from build123d import *

# Parameters (mm, degrees)
SKETCH_1_W             = 528
SKETCH_1_H             = 326
EXTRUDE_1_DEPTH        = 16
SKETCH_2_W             = 528
SKETCH_2_H             = 16
EXTRUDE_2_DEPTH        = 40
EXTRUDE_3_DEPTH        = 528
EXTRUDE_4_DEPTH        = 12
PATTERN_LINEAR_1_COUNT = 2
PATTERN_LINEAR_1_PITCH = 112
SKETCH_5_W             = 100
SKETCH_5_H             = 12
EXTRUDE_5_DEPTH        = 123
SKETCH_6_W             = 100
SKETCH_6_H             = 12
EXTRUDE_6_DEPTH        = 100
MIRROR_2_COPY_1_DEPTH  = 12


with BuildPart() as part:
    # 草图1 → 凸台-拉伸1 (new body)
    with BuildSketch(Plane(origin=(0, 0, 0), x_dir=(1, 0, 0), z_dir=(0, 1, 0))):
        Rectangle(SKETCH_1_W, SKETCH_1_H)
    extrude(amount=EXTRUDE_1_DEPTH)

    # 草图2 → 凸台-拉伸2 (add)
    with BuildSketch(Plane.XZ):
        with Locations((0, 145)):
            Rectangle(SKETCH_2_W, SKETCH_2_H)
        with Locations((0, -145)):
            Rectangle(SKETCH_2_W, SKETCH_2_H)
    extrude(amount=EXTRUDE_2_DEPTH)

    # 草图3 → 凸台-拉伸3 (add)
    with BuildSketch(Plane(origin=(264, 0, 0), x_dir=(0, 0, -1), z_dir=(1, 0, 0))):
        Polygon((-137, -40), (-137, 0), (137, 0), (137, -40), (132, -40), (132, -5), (-132, -5), (-132, -40), align=None)
    extrude(amount=-EXTRUDE_3_DEPTH)

    # 草图4 → 凸台-拉伸4 (add)
    with BuildSketch(Plane.ZY.offset(264)):
        with BuildLine():
            Line((-70, 139), (70, 139))
            ThreePointArc((70, 139), (91.213203436, 130.213203436), (100, 109))
            Line((100, 109), (100, 16))
            Line((100, 16), (-100, 16))
            Line((-100, 16), (-100, 109))
            ThreePointArc((-100, 109), (-91.213203436, 130.213203436), (-70, 139))
        make_face()
    extrude_4 = extrude(amount=-EXTRUDE_4_DEPTH)

    # 阵列(线性)1: 凸台-拉伸4 ×2
    with Locations(*[(i * PATTERN_LINEAR_1_PITCH, 0, 0) for i in range(1, PATTERN_LINEAR_1_COUNT)]):
        add(extrude_4)

    # 草图5 → 凸台-拉伸5 (add)
    with BuildSketch(Plane(origin=(0, 16, 0), x_dir=(1, 0, 0), z_dir=(0, 1, 0))):
        with Locations((-202, 56)):
            Rectangle(SKETCH_5_W, SKETCH_5_H)
        with Locations((-202, -56)):
            Rectangle(SKETCH_5_W, SKETCH_5_H)
    extrude_5 = extrude(amount=EXTRUDE_5_DEPTH)

    # 草图6 → 凸台-拉伸6 (add)
    with BuildSketch(Plane.ZY.offset(152)):
        with Locations((0, 89)):
            Rectangle(SKETCH_6_W, SKETCH_6_H)
    extrude_6 = extrude(amount=EXTRUDE_6_DEPTH)

    # 镜向2: 凸台-拉伸4, 凸台-拉伸5, 凸台-拉伸6 across plane
    add(extrude_4.mirror(Plane(origin=(0, 0, 0), x_dir=(0, 0, 1), z_dir=(1, 0, 0))))
    add(extrude_5.mirror(Plane(origin=(0, 0, 0), x_dir=(0, 0, 1), z_dir=(1, 0, 0))))
    add(extrude_6.mirror(Plane(origin=(0, 0, 0), x_dir=(0, 0, 1), z_dir=(1, 0, 0))))

    # 镜向2 copy 1 sketch → 镜向2 copy 1 (add)
    with BuildSketch(Plane(origin=(152, 0, 0), x_dir=(0, 0, 1), z_dir=(1, 0, 0))):
        with BuildLine():
            Line((-70, -139), (70, -139))
            ThreePointArc((70, -139), (91.213203436, -130.213203436), (100, -109))
            Line((100, -109), (100, -16))
            Line((100, -16), (-100, -16))
            Line((-100, -16), (-100, -109))
            ThreePointArc((-100, -109), (-91.213203436, -130.213203436), (-70, -139))
        make_face()
    extrude(amount=-MIRROR_2_COPY_1_DEPTH)


solid = part.part
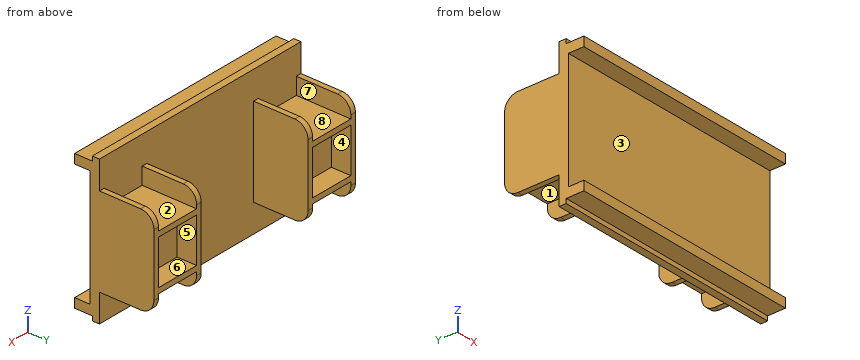
Verification items for the finished model (mm, model axes). Face numbers are marked on the shaded views. A direction names the side the tool comes from. Coordinates: 2 decimals unless noted, no trailing zeros. Order: outer loops, then holes, each group sorted by start corner. A loop starts at its lowest first (then second) coordinate and runs counter-clockwise, first axis right, second up. Notation, with made-up numbers: M -25.5,39.25 L 32.5,39.25 A6 cw 32.5,45.25 Z; hole C -27.5,-34 d3. An arc over 180 degrees is marked long. One line per item, written item: value. Start each with the question number.
Item 1: Depth check by flat-ended pin: P1, Ø10, axis at x = -14, z = -103.5, coming from the -Y side; P2, Ø1, axis at x = -154.5, y = 71, coming from the +Z side; P3, Ø6, axis at x = 256.5, y = 84, coming from the +Z side. Enter the tip coordinate at first touch or a pass-through.
Item 2: Thickness scan on probe 1 along X at (y, z) = (49, -69.5); probe 2 along X at (y, z) = (91, 39); probe 3 along Z at (x, y) = (15, -14). Record the ranges inside material, lowest first.
Item 3: Sectioned sample at D-D on x = -221.5. Record the cut outline in (y, z), then the cut area to 3 significant figures.
Item 4: Sectioned sample at B-B on y = -15.5. Record the cut outline in (x, z), then the cut area to 3 significant figures.
Item 5: Access from +Z, -Z, +X, -X, +Y, -Y to the whole of each face (thin tool, end or side, straight path). Record for the marked faces 1, 2, 3 and 4.
Item 6: Mould release check, pull along Z, two halves, no side actions. Record for the marked faces 5, 6, 7 and 8: pulls with the +Z half, pulls with the -Z half, needs draft (parallel to the pull), parting line crosses it, or undercut.
Item 7: Sectioned sample at A-A on y = 55.5. Give the number of separate pieces and of enclosed holes in the cut face, then the cut area to 3 significant figures.
Item 8: Sectioned sample at C-C on z = 15. Record the cut outline in (x, y), then the cut area to 3 significant figures.
Calculated:
1. P1: y = -5
1. P2: z = 62
1. P3: z = 100
2. probe 1: -264 to -252, -152 to -140, 140 to 152, 252 to 264
2. probe 2: -264 to -140, 140 to 264
2. probe 3: -153 to -132, 132 to 153
3. outline: M -40,-153 L 0,-153 L 0,-163 L 16,-163 L 16,-62 L 139,-62 L 139,-50 L 95,-50 L 95,50 L 139,50 L 139,62 L 16,62 L 16,163 L 0,163 L 0,153 L -40,153 L -40,132 L -5,132 L -5,-132 L -40,-132 Z; hole M 16,-50 L 83,-50 L 83,50 L 16,50 Z
3. area: 12,400 mm^2
4. outline: M -264,-153 L 264,-153 L 264,-132 L -264,-132 Z; M -264,132 L 264,132 L 264,153 L -264,153 Z
4. area: 22,200 mm^2
5. face 1: -Z, +Y
5. face 2: +Z, +Y
5. face 3: +X, -X, -Y
5. face 4: +Y
6. face 5: undercut
6. face 6: undercut
6. face 7: needs draft
6. face 8: pulls with the +Z half
7. separate pieces: 2
7. enclosed holes: 2
7. area: 14,400 mm^2
8. outline: M -264,-5 L 264,-5 L 264,139 L 252,139 L 252,95 L 152,95 L 152,139 L 140,139 L 140,16 L -140,16 L -140,139 L -152,139 L -152,95 L -252,95 L -252,139 L -264,139 Z; hole M -252,16 L -152,16 L -152,83 L -252,83 Z; hole M 152,16 L 252,16 L 252,83 L 152,83 Z
8. area: 19,400 mm^2
